Source: CAD feature listing. Evaluate the final solid. Frame: model axes, mm. Give positions to 0.01 mm unless a question says otherwise; leave off trailing zeros. Write each loop counter-clockwise with the first axis right and the second up, starting at its lowest first coordinate (ties: lowest second). Pieces come first, ordered by that corner, then holes. Notation, with made-up numbers: (41.5, -19.75) -> (72.5, -19.75) arc R24 cw to (72.5, 16.25) -> close; hole circle Ø2 at (9, -2.75). An arc over 180 degrees is marked (long way). Answer as a JSON object with one key per item and string values. Group by question number.
Item 1: Section query A-A on z = 206. Return the cut outline in (x, y).
Item 2: First-contact query: pin 1 Ø1 at (y, z) = (-1.5, 545) entering from +X; pin 2 Ø6.5 at (x, y) = (203, -4.5) entering from +Z; pin 3 Ø6.5 at (x, y) = (-182.5, -5) entering from +Z. Flat tips, straight axial feed; report the tip coordinate or a pass-through.
Item 3: Ray query, probe 1 along X at (y, z) = (-5, 102); probe 2 along Z at (x, y) = (-165.5, -3.5); probe 3 along Z at (x, y) = (167, -6.75). Return the intervals inside material, ascending. Write a range as from..to.
Item 4: Section query B-B on y = -8. Return the cut outline in (x, z), plus the area to 3 significant figures.
Item 5: Section query C-C on x = 34. Return the cut outline in (y, z), plus the area to 3 significant figures.
from build123d import *

# Parameters (mm, degrees)
F1_DEPTH = 12.7
F3_DEPTH = 12.701
F4_R     = 6.35
F5_R     = 25.4


with BuildPart() as f1:
    # F0 (on Front) → F1 (new body)
    with BuildSketch(Plane.XZ):
        Polygon((-304.8, 304.8), (-304.8, 0), (-144.824734, 0), (-144.824734, 38.1), (-271.824734, 38.1), (-271.824734, 241.3), (0, 241.3), (271.824734, 241.3), (271.824734, 38.1), (144.824734, 38.1), (144.824734, 0), (304.8, 0), (304.8, 304.8), (0, 609.6), align=None)
    extrude(amount=F1_DEPTH)

    # F2 (on Front) → F3 (cut, through all)
    with BuildSketch(Plane.XZ):
        Polygon((0, 532.894433), (-245.717928, 298.267931), (231.313556, 290.646062), align=None)
    extrude(amount=F3_DEPTH, mode=Mode.SUBTRACT)

    # F4
    f4_edges = [f1.edges().sort_by_distance(p)[0] for p in [
        (0, -6.35, 609.6),
    ]]
    fillet(f4_edges, radius=F4_R)

    # F5
    f5_edges = [f1.edges().sort_by_distance(p)[0] for p in [
        (-271.824734, -6.35, 38.1),
        (-271.824734, -6.35, 241.3),
        (271.824734, -6.35, 241.3),
        (271.824734, -6.35, 38.1),
        (-245.717928, -6.35, 298.267931),
        (231.313556, -6.35, 290.646062),
        (0, -6.35, 532.894433),
    ]]
    fillet(f5_edges, radius=F5_R)


solid = f1.part
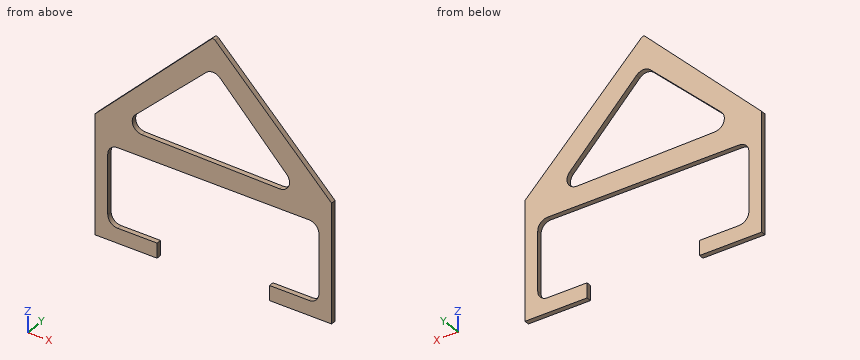
Worked answers:
{
 "1": {"outline": "(-304.8, -12.7) -> (-271.82, -12.7) -> (-271.82, 0) -> (-304.8, 0) -> close; (271.82, -12.7) -> (304.8, -12.7) -> (304.8, 0) -> (271.82, 0) -> close"},
 "2": {"pin 1": "x = 65.1", "pin 2": "z = 409.85", "pin 3": "z = 430.35"},
 "3": {"probe 1": "-304.8..-271.82, 271.82..304.8", "probe 2": "0..38.1, 241.3..296.99, 374.86..444.1", "probe 3": "0..38.1, 241.3..291.67, 358..442.6"},
 "4": {"outline": "(-304.8, 0) -> (-144.82, 0) -> (-144.82, 38.1) -> (-246.42, 38.1) arc R25.4 cw to (-271.82, 63.5) -> (-271.82, 215.9) arc R25.4 cw to (-246.42, 241.3) -> (246.42, 241.3) arc R25.4 cw to (271.82, 215.9) -> (271.82, 63.5) arc R25.4 cw to (246.42, 38.1) -> (144.82, 38.1) -> (144.82, 0) -> (304.8, 0) -> (304.8, 304.8) -> (4.49, 605.11) arc R6.35 ccw to (-4.49, 605.11) -> (-304.8, 304.8) -> close; hole (-200.92, 341.05) arc R25.4 ccw to (-183.78, 297.28) -> (170.61, 291.62) arc R25.4 ccw to (189.39, 334.55) -> (17.54, 514.52) arc R25.4 ccw to (-18.37, 515.35) -> close", "area": "103,000 mm^2"},
 "5": {"outline": "(-12.7, 241.3) -> (0, 241.3) -> (0, 293.8) -> (-12.7, 293.8) -> close; (-12.7, 497.29) -> (0, 497.29) -> (0, 575.6) -> (-12.7, 575.6) -> close", "area": "1,660 mm^2"}
}
